Verification items for the finished model (mm, model axes). A direction names the side the tool comes from. Give positions to 0.01 mm unless a question says otherwise; leave off trailing zeros. Write each loop counter-clockwise with the first axis right and the second up, starting at its lowest first coordinate (ties: lowest second). Pieces come first, ordered by that corner, then holes.
from build123d import *
from build123d.topology import SkipClean

# Parameters (mm, degrees)
SKETCH_5_W                 = 17
SKETCH_5_H                 = 100
EXTRUDE_1_DEPTH            = 15
PATTERN_LINEAR_1_COUNT     = 2
PATTERN_LINEAR_1_PITCH     = 16.1
PATTERN_LINEAR_1_COL_COUNT = 2
PATTERN_LINEAR_1_COL_PITCH = 16.1
SKETCH_8_W                 = 8
SKETCH_8_H                 = 22
SKETCH_9_W                 = 55
SKETCH_9_H                 = 5


with BuildPart() as part:
    # Sketch 5 → Extrude 1 (new, symmetric)
    with BuildSketch(Plane.XY):
        with Locations((-8.5, 20)):
            Rectangle(SKETCH_5_W, SKETCH_5_H)
    extrude_1 = extrude(amount=EXTRUDE_1_DEPTH, both=True)

    # Sketch 7 → Cut-Revolve 1 (revolve, cut)
    with BuildSketch(Plane.XY):
        with BuildLine():
            Line((-17, 5), (-17, -11))
            ThreePointArc((-17, -11), (-9, -3), (-17, 5))
        make_face()
    cut_revolve_1 = revolve(axis=Axis((-17, 5, 0), (0, -1, 0)), mode=Mode.SUBTRACT)

    # Pattern Linear 1: Cut-Revolve 1 ×2
    with Locations(*[(0, i * PATTERN_LINEAR_1_PITCH, 0) for i in range(1, PATTERN_LINEAR_1_COUNT)]):
        add(cut_revolve_1, mode=Mode.SUBTRACT)

    # Pattern Linear 1 col: Cut-Revolve 1 ×2
    with Locations(*[(0, -i * PATTERN_LINEAR_1_COL_PITCH, 0) for i in range(1, PATTERN_LINEAR_1_COL_COUNT)]):
        add(cut_revolve_1, mode=Mode.SUBTRACT)

    # Mirror 2: Extrude 1 across plane
    add(extrude_1.mirror(Plane(origin=(0, 0, 0), x_dir=(0, 0, 1), z_dir=(1, 0, 0))))

    # Mirror 3: Cut-Revolve 1 across plane
    with SkipClean():  # the faces are left unmerged after this step: merging them gives an invalid solid
        add(cut_revolve_1.mirror(Plane(origin=(0, 0, 0), x_dir=(0, 0, 1), z_dir=(1, 0, 0))), mode=Mode.SUBTRACT)

    # Mirror 4 copy 1 sketch → Mirror 4 copy 1 (revolve, cut)
    with SkipClean():  # the faces are left unmerged after this step: merging them gives an invalid solid
        with BuildSketch(Plane(origin=(0, 16.1, 0), x_dir=(-1, 0, 0), z_dir=(0, 0, 1))):
            with BuildLine():
                Line((-17, -5), (-17, 11))
                ThreePointArc((-17, 11), (-9, 3), (-17, -5))
            make_face()
        revolve(axis=Axis((17, 21.1, 0), (0, 1, 0)), mode=Mode.SUBTRACT)

    # Mirror 4 copy 2 sketch → Mirror 4 copy 2 (revolve, cut)
    with SkipClean():  # the faces are left unmerged after this step: merging them gives an invalid solid
        with BuildSketch(Plane(origin=(0, -16.1, 0), x_dir=(-1, 0, 0), z_dir=(0, 0, 1))):
            with BuildLine():
                Line((-17, -5), (-17, 11))
                ThreePointArc((-17, 11), (-9, 3), (-17, -5))
            make_face()
        revolve(axis=Axis((17, -11.1, 0), (0, 1, 0)), mode=Mode.SUBTRACT)

    # Mirror 4 copy 3 sketch → Mirror 4 copy 3 (revolve, cut)
    with SkipClean():  # the faces are left unmerged after this step: merging them gives an invalid solid
        with BuildSketch(Plane(origin=(0, 0, 0), x_dir=(-1, 0, 0), z_dir=(0, 0, 1))):
            with BuildLine():
                Line((-17, -5), (-17, 11))
                ThreePointArc((-17, 11), (-9, 3), (-17, -5))
            make_face()
        revolve(axis=Axis((17, 5, 0), (0, 1, 0)), mode=Mode.SUBTRACT)

    # Sketch 8 → Cut-Revolve 2 (revolve, cut)
    with SkipClean():  # the faces are left unmerged after this step: merging them gives an invalid solid
        with BuildSketch(Plane.XY):
            with Locations((-4, -19)):
                Rectangle(SKETCH_8_W, SKETCH_8_H)
        revolve(axis=Axis((0, -8, 0), (0, -1, 0)), mode=Mode.SUBTRACT)

    # Sketch 9 → Revolve 1 (revolve)
    with SkipClean():  # the faces are left unmerged after this step: merging them gives an invalid solid
        with BuildSketch(Plane.XY, mode=Mode.PRIVATE) as revolve_1_sk:
            with Locations((27.5, 72.5)):
                Rectangle(SKETCH_9_W, SKETCH_9_H)
        revolve(revolve_1_sk.sketch.rotate(Axis((0, 70, 0), (0, 1, 0)), 90), axis=Axis((0, 70, 0), (0, 1, 0)))


solid = part.part
Item 1: Release check for a two-part mould opening along Z. For faces 6 (the face through (-17, 30, 0)), 7 (the face through (0, -8, 0)), 8 (the face through (1.73, -18.85, 7.81)), 9 (the face through (48.794, 72.535, -25.379)) record: released by +Z, released by -Z, zero draft, split by the parting line, or undercut.
Answer key:
face 6: zero draft
face 7: undercut
face 8: undercut
face 9: split by the parting line
Item 2: Set-up check for faces 1 (the face through (8, -30, 4)), 2 (the face through (0, 21, 15)), 3 (the face through (-1, 75, -1)), 4 (the face through (17, 30, 0)), 5 (the face through (0, 21, -15)): record each of +Z, -Z, +X, -X, +Y, -Y from which the full face is reachable in a straight line by a thin tool's end or side.
Answer key:
face 1: +Z, -Z, +X, -X, -Y
face 2: +Z, +X, -X, -Y
face 3: +Z, -Z, +X, -X, +Y
face 4: +Z, -Z, +X, -Y
face 5: -Z, +X, -X, -Y
Item 3: Depth check by flat-ended pin: pin 1 (8 mm diameter, centred on x = -2.5, z = 3, fed in from -Y); pin 2 (8 mm diameter, centred on y = -7, z = 3, fed in from +X); pin 3 (10 mm diameter, centred on x = 40.5, z = -32, fed in from -Y). Enter the tip coordinate at first touch or a pass-through.
Answer key:
pin 1: stops at y = -8
pin 2: stops at x = 17
pin 3: stops at y = 70
Item 4: Sectioned sample at B-B on y = -22. Record the cut outline in (x, z).
Answer key:
outline: (-17, -15) - (17, -15) - (17, -7.46) arc R7.46 cw to (17, 7.46) - (17, 15) - (-17, 15) - (-17, 7.46) arc R7.46 cw to (-17, -7.46) - close; hole circle Ø16 at (0, 0)
Item 5: Scan lines: line 1 along Z through (x, y) = (0, -21.75); line 2 along Y through (x, z) = (15, 30); line 3 along X through (y, z) = (-18.25, 0). Record each from-to range of solid material in increasing order.
Answer key:
line 1: z = -15 to -8, 8 to 15
line 2: y = 70 to 75
line 3: x = -9.05 to -8, 8 to 9.05
Item 6: Sectioned sample at C-C on z = -10.5. Record the cut outline in (x, y).
Answer key:
outline: (-53.99, 70) - (-17, 70) - (-17, -30) - (17, -30) - (17, 70) - (53.99, 70) - (53.99, 75) - (-53.99, 75) - close
Item 7: Sectioned sample at A-A on x = 0. Record the cut outline in (y, z), then the cut area to 3 significant figures.
Answer key:
outline: (-30, -15) - (70, -15) - (70, -55) - (75, -55) - (75, 55) - (70, 55) - (70, 15) - (-30, 15) - (-30, 8) - (-8, 8) - (-8, -8) - (-30, -8) - close
area: 3,200 mm2
Item 8: Sectioned sample at D-D on y = 49.5. Record the cut outline in (x, z).
Answer key:
outline: (-17, -15) - (17, -15) - (17, 15) - (-17, 15) - close
